Build history of the part. All positions in model axes, mm. Round coordinates to 2 decimals unless told otherwise and drop trailing zeros. Write each loop counter-clockwise with the first axis right and the second up, starting at its lowest first coordinate (ties: lowest second). Pieces come first, ordered by that corner, then holes. Notation, with made-up numbers: (7.25, 0.25) -> (30.25, 0.25) arc R20 cw to (30.25, 29.25) -> close; hole circle Ø1 at (-30.75, -32.5). An arc over 180 degrees is marked (long way). Answer in a Markdown table with one row per item.
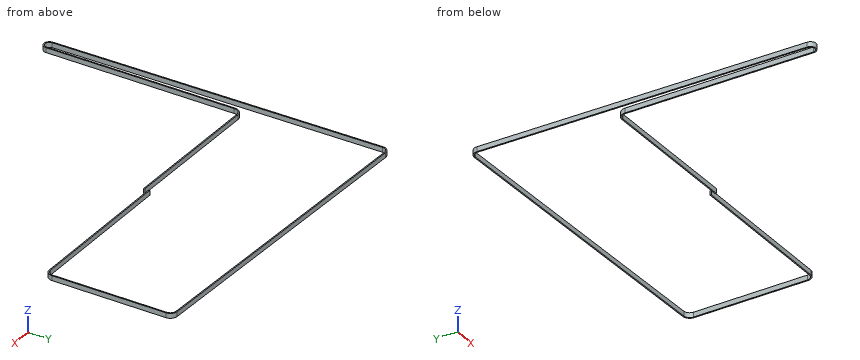
```python
from build123d import *

# Parameters (mm, degrees)
EXTRUDE_1_DEPTH = 6


with BuildPart() as part:
    # Эскиз1 → Вытянуть-Тонкостенный1 (new body)
    with BuildSketch(Plane.XY):
        with BuildLine():
            Line((199.171010966, 244.669379092), (15.850409713, 244.973028732))
            ThreePointArc((15.850409713, 244.973028732), (9.76523397, 242.3635414), (7.250012003, 236.238800882))
            Line((7.250012003, 236.238800882), (6.858690591, -0.011360638))
            ThreePointArc((6.858690591, -0.011360638), (0.022547579, -6.858662938), (-6.858467649, -0.056455245))
            Line((-6.858467649, -0.056455245), (-10.249703578, 411.927977114))
            ThreePointArc((-10.249703578, 411.927977114), (-7.648126176, 418.225997476), (-1.317862082, 420.748104128))
            Line((-1.317862082, 420.748104128), (396.829346884, 412.458570479))
            ThreePointArc((396.829346884, 412.458570479), (402.912249078, 409.818802658), (405.397119956, 403.670998988))
            Line((405.397119956, 403.670998988), (404.749910989, 260.184840159))
            ThreePointArc((404.749910989, 260.184840159), (402.225998422, 254.076182312), (396.149590287, 251.475586319))
            Line((396.149590287, 251.475586319), (199.120398676, 250.818015146))
            Line((199.120398676, 250.818015146), (199.115392559, 252.318006792))
            Line((199.115392559, 252.318006792), (396.13377965, 252.975541906))
            ThreePointArc((396.13377965, 252.975541906), (401.162138455, 255.133646805), (403.249926248, 260.191605993))
            Line((403.249926248, 260.191605993), (403.897135215, 403.677764822))
            ThreePointArc((403.897135215, 403.677764822), (401.838242202, 408.771659292), (396.798123241, 410.958895487))
            Line((396.798123241, 410.958895487), (-1.349085725, 419.248429135))
            ThreePointArc((-1.349085725, 419.248429135), (-6.594161688, 417.158683623), (-8.749754393, 411.940323895))
            Line((-8.749754393, 411.940323895), (-5.358518464, -0.044108464))
            ThreePointArc((-5.358518464, -0.044108464), (0.017616416, -5.358671043), (5.358692649, -0.008876062))
            Line((5.358692649, -0.008876062), (5.750014061, 236.241285457))
            ThreePointArc((5.750014061, 236.241285457), (8.70154817, 243.421188856), (15.839385081, 246.473049051))
            Line((15.839385081, 246.473049051), (199.173495541, 246.169377034))
            Line((199.173495541, 246.169377034), (199.171010966, 244.669379092))
        make_face()
    extrude(amount=EXTRUDE_1_DEPTH)


solid = part.part
```
Q1. Drop flat-ended pins along their axis: P1, Ø2, axis at y = 279.5, z = 5, coming from the -X side; P2, Ø3, axis at y = 342.5, z = 3, coming from the -X side; P3, Ø3, axis at x = 300, z = 3, coming from the -Y side. Give the stop position or say it passes through.
A:
| item | result |
|---|---|
| P1 | x = -9.17 |
| P2 | x = -9.69 |
| P3 | y = 251.15 |
Q2. Saw through at A-A on x = 347. Write the cut outline in (y, z).
A:
| item | result |
|---|---|
| outline | (251.31, 0) -> (252.81, 0) -> (252.81, 6) -> (251.31, 6) -> close; (412, 0) -> (413.5, 0) -> (413.5, 6) -> (412, 6) -> close |
Q3. Wall check: line 1 (Y direction, x = 250.5, z = 3.45); line 2 (Y direction, x = 246.5, z = 1.95); line 3 (X direction, y = 159, z = 1.2). Give the ranges that are in metal, low to high. Write a range as [from, to].
A:
| item | result |
|---|---|
| line 1 | [250.99, 252.49], [414, 415.51] |
| line 2 | [250.98, 252.48], [414.09, 415.59] |
| line 3 | [-8.17, -6.67], [5.62, 7.12] |
Q4. Saw through at C-C on z = 5.05. Write the cut outline in (x, y), plus the area to 3 significant figures.
A:
| item | result |
|---|---|
| outline | (-10.25, 411.93) -> (-6.86, -0.06) arc R6.86 ccw to (6.86, -0.01) -> (7.25, 236.24) arc R8.75 cw to (15.85, 244.97) -> (199.17, 244.67) -> (199.17, 246.17) -> (15.84, 246.47) arc R10.25 ccw to (5.75, 236.24) -> (5.36, -0.01) arc R5.36 cw to (-5.36, -0.04) -> (-8.75, 411.94) arc R7.25 cw to (-1.35, 419.25) -> (396.8, 410.96) arc R7.25 cw to (403.9, 403.68) -> (403.25, 260.19) arc R7.25 cw to (396.13, 252.98) -> (199.12, 252.32) -> (199.12, 250.82) -> (396.15, 251.48) arc R8.75 ccw to (404.75, 260.18) -> (405.4, 403.67) arc R8.75 ccw to (396.83, 412.46) -> (-1.32, 420.75) arc R8.75 ccw to start |
| area | 2,460 mm² |
Q5. Saw through at B-B on y = 56.5. Write the cut outline in (x, z), plus the area to 3 significant figures.
A:
| item | result |
|---|---|
| outline | (-7.32, 0) -> (-5.82, 0) -> (-5.82, 6) -> (-7.32, 6) -> close; (5.45, 0) -> (6.95, 0) -> (6.95, 6) -> (5.45, 6) -> close |
| area | 18.0 mm² |
